```python
from build123d import *

# Parameters (mm, degrees)
EXTRUDE1_DEPTH  = 820
LPATTERN1_COUNT = 14
LPATTERN1_PITCH = 60


with BuildPart() as part:
    # Sketch1 → Extrude1 (new body)
    with BuildSketch(Plane(origin=(-20, 0, 0), x_dir=(1, 0, 0), z_dir=(0, 0, 1))):
        with BuildLine():
            Line((12.5, 0.69999271), (13.199992786, 0))
            Line((13.199992786, 0), (26.800007214, 0))
            Line((26.800007214, 0), (27.5, 0.69999271))
            Line((27.5, 0.69999271), (27.5, 4.2000246))
            Line((27.5, 4.2000246), (24.8000183, 6.9000063))
            Line((24.8000183, 6.9000063), (24.8000183, 8.8400054))
            Line((24.8000183, 8.8400054), (25.755946813, 9.794179118))
            ThreePointArc((25.755946813, 9.794179118), (26.198484624, 10.690600567), (27.09432569, 11.13431209))
            Line((27.09432569, 11.13431209), (27.5, 11.5399866))
            Line((27.5, 11.5399866), (27.5, 12.8500204))
            Line((27.5, 12.8500204), (27.09432569, 13.268442751))
            ThreePointArc((27.09432569, 13.268442751), (26.202460867, 13.706434947), (25.755946813, 14.594063938))
            Line((25.755946813, 14.594063938), (25.3500197, 15))
            Line((25.3500197, 15), (14.6499803, 15))
            Line((14.6499803, 15), (14.244053187, 14.594063938))
            ThreePointArc((14.244053187, 14.594063938), (13.797539133, 13.706434947), (12.90567431, 13.268442751))
            Line((12.90567431, 13.268442751), (12.5, 12.8500204))
            Line((12.5, 12.8500204), (12.5, 11.5399866))
            Line((12.5, 11.5399866), (12.90567431, 11.13431209))
            ThreePointArc((12.90567431, 11.13431209), (13.801515376, 10.690600567), (14.244053187, 9.794179118))
            Line((14.244053187, 9.794179118), (15.1999817, 8.8400054))
            Line((15.1999817, 8.8400054), (15.1999817, 6.9000063))
            Line((15.1999817, 6.9000063), (12.5, 4.2000246))
            Line((12.5, 4.2000246), (12.5, 0.69999271))
        make_face()
    extrude(amount=-EXTRUDE1_DEPTH)

    # Sketch2 → Cut-Revolve1 (revolve, cut)
    with BuildSketch(Plane(origin=(0, 0, 0), x_dir=(0, 0, -1), z_dir=(1, 0, 0)), mode=Mode.PRIVATE) as cut_revolve1_sk:
        Polygon((20, 15), (23.75, 15), (23.75, 9.7), (22.25, 9.7), (22.25, 0), (20, 0), align=None)
    cut_revolve1 = revolve(cut_revolve1_sk.sketch.rotate(Axis((0, 0, -20), (0, 1, 0)), 180), axis=Axis((0, 0, -20), (0, 1, 0)), mode=Mode.SUBTRACT)

    # LPattern1: Cut-Revolve1 ×14
    with Locations(*[(0, 0, -i * LPATTERN1_PITCH) for i in range(1, LPATTERN1_COUNT)]):
        add(cut_revolve1, mode=Mode.SUBTRACT)


solid = part.part
```
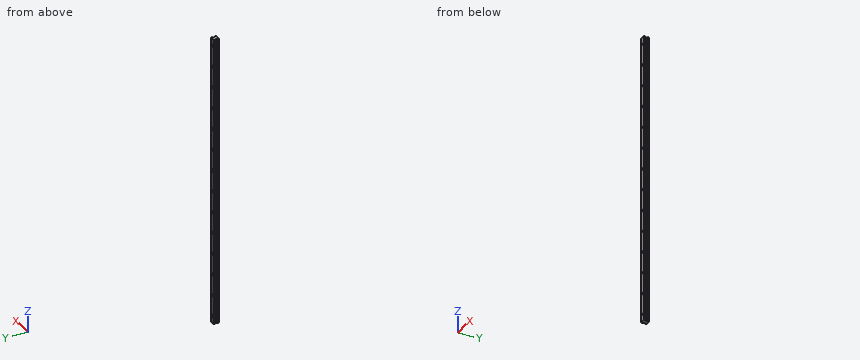
Geometry check sheet. Reference: the model listing, model coordinates, mm. Round coordinates to 2 decimals unless told otherwise and drop trailing zeros. Loops run counter-clockwise (first coordinate to the right, second up) from the corner with the lowest first, then second, coordinate; pieces in that order, holes last. Notation, with made-up numbers: M -20.75,-2 L -4.75,-2 A23 cw -4.75,28 Z; hole C 42.5,27.25 d3. An arc over 180 degrees is marked long. Return JSON: item names as keys, results as strings. Group by question number.
(1) Go/stop test with flat-tipped pins: pin 1 (3 mm diameter, centred on y = 7, z = -144.5, fed in from -X); pin 2 (6 mm diameter, centred on y = 8, z = -359.5, fed in from +X); pin 3 (7 mm diameter, centred on x = 0, z = -800, fed in from +Y). Record where each tip stops, or that it passes through.
(2) Scan lines: line 1 along X through (y, z) = (6.75, -560); line 2 along X through (y, z) = (12.9, -20); line 3 along Y through (x, z) = (6.25, -407). Record each from-to range of solid material in increasing order. Write a range as [from, to].
(3) Section check B-B, the plane x = 0. Give the number of separate pieces and of enclosed holes in the cut face, and give its area (3 significant figures).
(4) Section check A-A, the plane z = -477.5. Enter the section's corners in (x, y), and give its area (3 significant figures).
Data:
{
 "1": {"pin 1": "x = -6.2", "pin 2": "x = 6.7", "pin 3": "y = 9.7"},
 "2": {"line 1": "[-4.95, -2.25], [2.25, 4.95]", "line 2": "[-7.45, -3.75], [3.75, 7.45]", "line 3": "[0, 5.45], [10.74, 13.66]"},
 "3": {"separate pieces": "15", "enclosed holes": "0", "area": "11,100 mm²"},
 "4": {"outline": "M -7.5,0.7 L -6.8,0 L 6.8,0 L 7.5,0.7 L 7.5,4.2 L 4.8,6.9 L 4.8,8.84 L 5.76,9.79 A1.56 cw 7.09,11.13 L 7.5,11.54 L 7.5,12.85 L 7.09,13.27 A1.56 cw 5.76,14.59 L 5.35,15 L -5.35,15 L -5.76,14.59 A1.56 cw -7.09,13.27 L -7.5,12.85 L -7.5,11.54 L -7.09,11.13 A1.56 cw -5.76,9.79 L -4.8,8.84 L -4.8,6.9 L -7.5,4.2 Z", "area": "193 mm²"}
}
